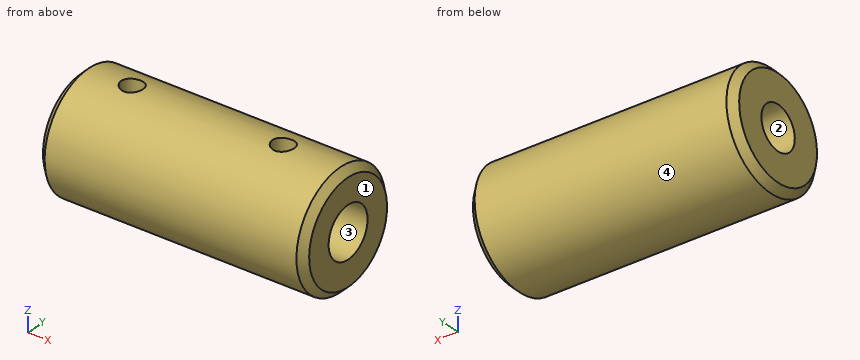
from build123d import *

# Parameters (mm, degrees)
ESBO_O2_R             = 1.5
CORTE_EXTRUS_O1_DEPTH = 121.149937162


with BuildPart() as part:
    # Esboço1 → Revolução1 (revolve)
    with BuildSketch(Plane.XY, mode=Mode.PRIVATE) as revolu_o1_sk:
        Polygon((81.95, -3.93), (81.95, 0.07), (82.95, 1.07), (117.95, 1.07), (118.95, 0.07), (118.95, -3.43), (102.7, -3.43), (101.7, -3.93), (101.7, -6.93), (97.95, -6.93), (97.95, -4.93), (96.95, -3.93), align=None)
    revolve(revolu_o1_sk.sketch.rotate(Axis((81.95, -6.93, 0), (1, 0, 0)), 90), axis=Axis((81.95, -6.93, 0), (1, 0, 0)))

    # Esboço2 → Corte-extrusão1 (cut, through all)
    with BuildSketch(Plane.XY):
        with Locations(Location((88.95, -6.93, 0), (0, 0, 180))):
            Circle(ESBO_O2_R)
        with Locations(Location((109.95, -6.93, 0), (0, 0, 180))):
            Circle(ESBO_O2_R)
    extrude(amount=CORTE_EXTRUS_O1_DEPTH, mode=Mode.SUBTRACT)


solid = part.part
Part model, mm, in its own coordinate system. Face numbers are marked on the shaded views. Coordinates: 2 decimals unless noted, no trailing zeros. Order: outer loops, then holes, each group sorted by start corner. A loop starts at its lowest first (then second) coordinate and runs counter-clockwise, first axis right, second up. Notation, with made-up numbers: M 18,12.25 L 71,12.25 A20 ccw 71,39.25 Z; hole C -9,51 d3. An arc over 180 degrees is marked long. One line per question, with ' | ' between items.
Q1. Pin check, flat tips, straight feed: P1, Ø1, axis at x = 92, y = -12, coming from the -Z side; P2, Ø3, axis at y = -8, z = 0.5, coming from the -X side; P3, Ø1.5, axis at x = 90, y = -11, coming from the -Z side. Stop position of each tip, or through.
A:
P1: stops at z = -6.57 | P2: stops at x = 97.27 | P3: stops at z = -7.28
Q2. Two-plate mould, pull along Z, no slides. Class the marked faces 1, 2, 3 and 4: +Z half, -Z half, draft (parallel to the pull), parting line (faces both ways), or undercut.
A:
face 1: draft | face 2: undercut | face 3: undercut | face 4: parting line
Q3. Slice it at A-A (y = -6.93). Give the cut face in (x, z), and give its area (3 significant figures).
A:
outline: M 81.95,-7 L 82.95,-8 L 117.95,-8 L 118.95,-7 L 118.95,-3.5 L 102.7,-3.5 L 101.7,-3 L 101.7,3 L 102.7,3.5 L 108.45,3.5 L 108.45,8 L 90.45,8 L 90.45,3 L 96.95,3 L 97.95,2 L 97.95,-2 L 96.95,-3 L 81.95,-3 Z; M 81.95,3 L 87.45,3 L 87.45,8 L 82.95,8 L 81.95,7 Z; M 111.45,3.5 L 118.95,3.5 L 118.95,7 L 117.95,8 L 111.45,8 Z | area: 346 mm^2
Q4. Slice it at B-B (z = 0). Give the cut face in (x, y), and give its area (3 significant figures).
A:
outline: M 81.95,-13.93 L 82.95,-14.93 L 117.95,-14.93 L 118.95,-13.93 L 118.95,-10.43 L 102.7,-10.43 L 101.7,-9.93 L 101.7,-3.93 L 102.7,-3.43 L 118.95,-3.43 L 118.95,0.07 L 117.95,1.07 L 82.95,1.07 L 81.95,0.07 L 81.95,-3.93 L 96.95,-3.93 L 97.95,-4.93 L 97.95,-8.93 L 96.95,-9.93 L 81.95,-9.93 Z | area: 375 mm^2
Q5. Slice it at C-C (x = 93). Give the cut face in (y, z), and give its area (3 significant figures).
A:
outline: C -6.93,0 d16; hole C -6.93,0 d6 | area: 173 mm^2
Q6. Drill centre lines: line 1 (Y direction, x = 88, z = 0); line 2 (X direction, y = -7.75, z = 1.75); line 3 (Z direction, x = 103.5, y = -4.75). Where is each one in solid material? Low to high.
A:
line 1: y = -14.93 to -9.93, -3.93 to 1.07 | line 2: x = 97.95 to 101.7 | line 3: z = -7.7 to -2.74, 2.74 to 7.7
Q7. Slice it at D-D (z = 5.5). Count the separate pieces of the cut face and the enclosed holes in it, and give its area (3 significant figures).
A:
separate pieces: 1 | enclosed holes: 2 | area: 413 mm^2
